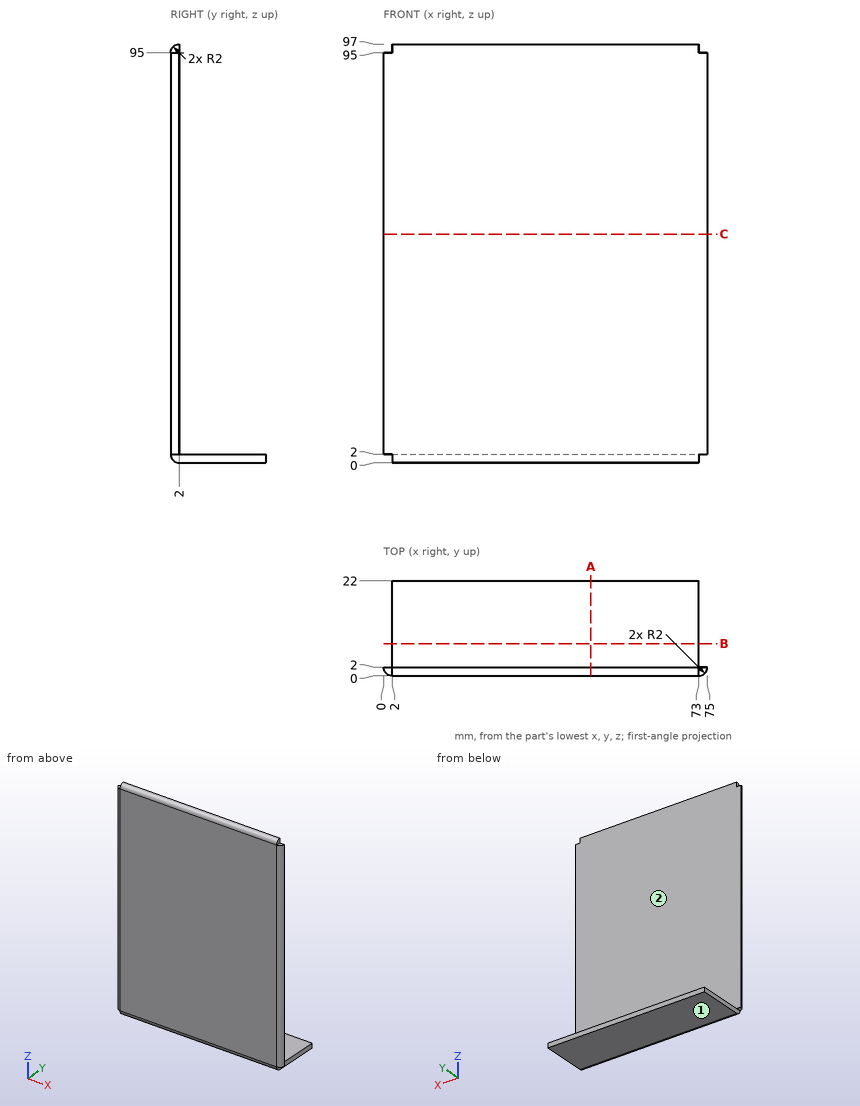
Can you work these out from the drawing? Everything is in mm from the part's minimum corner. A direction names the side the tool comes from. Round coordinates to 2 decimals unless told otherwise and drop trailing zeros. Order: outer loops, then holes, each group sorted by start corner. A loop starts at its lowest first (then second) coordinate and runs counter-clockwise, first axis right, second up. Notation, with made-up numbers: (78, 23) -> (137, 23) arc R22 cw to (137, 54) -> close; hole circle Ø3 at (72.5, 44). An arc over 180 degrees is marked (long way). Return JSON: item names as keys, results as strings. Group by question number.
1. I need wall thicknesses on line 1 (Y direction, x = 34.5, z = 45). Which ranges of the line are inside material? Lowest first, please. Write a range as [from, to].
2. If we section it at A-A, the plane x = 48: Write out the boundary of the cut face in (y, z), then the cut area to 3 significant figures.
3. If we section it at B-B, the plane y = 7.5: Write out the boundary of the cut face in (x, z).
4. Will these pins go through, and if not, where does the flat tip stop? pin 1 (1.6 mm diameter, centred on y = 11, z = 0.5, fed in from -X); pin 2 (8 mm diameter, centred on y = 9.5, z = 72.5, fed in from -X); pin 3 (1.6 mm diameter, centred on y = 16.5, z = 0.5, fed in from +X); pin 4 (6 mm diameter, centred on x = 47, y = 7.5, fed in from +Z).
5. Which directions (+Z, -Z, +X, -X, +Y, -Y) give clear straight access to the entire face, cutting with the end or side of a thin tool? Please do the marked faces 1 and 2.
6. If we section it at C-C, the plane z = 53: Write out the boundary of the cut face in (x, y).
Output values:
{
 "1": {"line 1": "[0, 2]"},
 "2": {"outline": "(0, 2) arc R2 ccw to (2, 0) -> (22, 0) -> (22, 2) -> (2, 2) -> (2, 97) arc R2 ccw to (0, 95) -> close", "area": "232 mm²"},
 "3": {"outline": "(2, 0) -> (73, 0) -> (73, 2) -> (2, 2) -> close"},
 "4": {"pin 1": "x = 2", "pin 2": "through", "pin 3": "x = 73", "pin 4": "z = 2"},
 "5": {"face 1": "-Z, +X, -X, +Y, -Y", "face 2": "+Z, +X, -X, +Y"},
 "6": {"outline": "(0, 2) arc R2 ccw to (2, 0) -> (73, 0) arc R2 ccw to (75, 2) -> close"}
}
